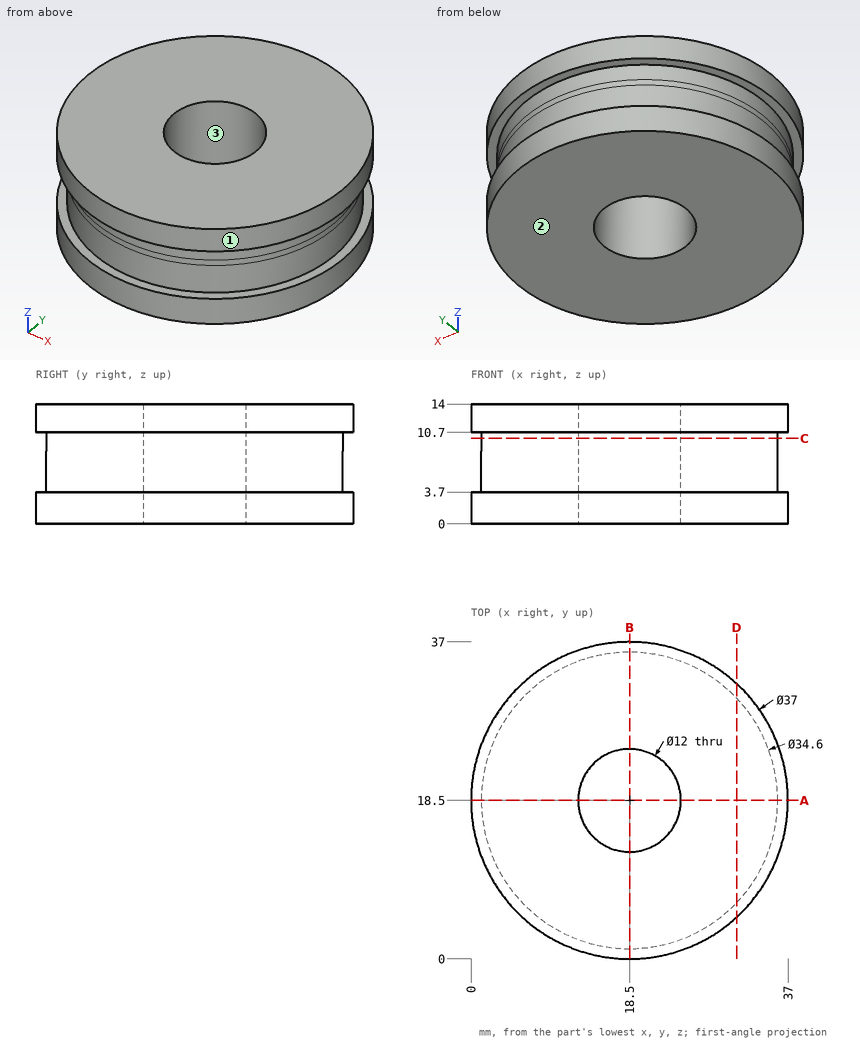
Print and shaded views of the part. All mm, measured from the part's lowest x, y and z. Give positions to 0.01 mm unless a question says otherwise; leave off trailing zeros. Loops run counter-clockwise (first coordinate to the right, second up) from the corner with the lowest first, then second, coordinate; pieces in that order, holes last. Notation, with made-up numbers: (56.5, 36.25) - (61.5, 36.25) arc R17 ccw to (61.5, 44.25) - close; hole circle Ø1 at (51.5, -11.75). An arc over 180 degrees is marked (long way). Use a Markdown table: item, result.
(1) Band-saw the part on A-A (y = 18.5). Give the cut face in (x, z).
Taken from the geometry:
| item | result |
|---|---|
| outline | (0, 0) - (12.5, 0) - (12.5, 14) - (0, 14) - (0, 10.7) - (1.2, 10.7) - (1.2, 3.7) - (0, 3.7) - close; (24.5, 0) - (37, 0) - (37, 3.7) - (35.8, 3.7) - (35.8, 10.7) - (37, 10.7) - (37, 14) - (24.5, 14) - close |
(2) Band-saw the part on C-C (z = 10). Give the cut face in (x, y), and give its area (3 significant figures).
Taken from the geometry:
| item | result |
|---|---|
| outline | circle Ø34.6 at (18.5, 18.5); hole circle Ø12 at (18.5, 18.5) |
| area | 827 mm2 |
(3) Drop flat-ended pins along their axis: pin 1 Ø8 at (y, z) = (11.5, 3) entering from +X; pin 2 Ø2 at (x, z) = (31.5, 12) entering from +Y; pin 3 Ø4 at (x, z) = (29.5, 11.5) entering from -Y. Give the stop position or say it passes through.
Taken from the geometry:
| item | result |
|---|---|
| pin 1 | x = 36.76 |
| pin 2 | y = 32.58 |
| pin 3 | y = 2.34 |
(4) Band-saw the part on D-D (x = 31). Give the cut face in (y, z), and give its area (3 significant figures).
Taken from the geometry:
| item | result |
|---|---|
| outline | (4.86, 0) - (32.14, 0) - (32.14, 3.7) - (30.46, 3.7) - (30.46, 10.7) - (32.14, 10.7) - (32.14, 14) - (4.86, 14) - (4.86, 10.7) - (6.54, 10.7) - (6.54, 3.7) - (4.86, 3.7) - close |
| area | 358 mm2 |
(5) Wall check: line 1 along Y through (x, z) = (18.5, 7.25); line 2 along Y through (x, z) = (18.5, 3.25); line 3 along X through (y, z) = (22.5, 6). Give the ranges that are in metal, low to high.
Taken from the geometry:
| item | result |
|---|---|
| line 1 | 1.2 to 12.5, 24.5 to 35.8 |
| line 2 | 0 to 12.5, 24.5 to 37 |
| line 3 | 1.67 to 14.03, 22.97 to 35.33 |
(6) Pull direction Y, two halves, no side cores. Call the marked faces 1, 2 and 3: +Y half, -Y half, draft (parallel to the pull), parting line (faces both ways), or undercut.
Taken from the geometry:
| item | result |
|---|---|
| face 1 | parting line |
| face 2 | draft |
| face 3 | undercut |
